Can you work these out from the model? Positions are in its coordinate system, mm. Face numbers are marked on the shaded views. A direction names the side the tool comes from. Give positions to 0.01 mm unless a question says otherwise; leave off trailing zeros. Loops run counter-clockwise (first coordinate to the right, second up) from the corner with the lowest first, then second, coordinate; pieces in that order, holes last. Notation, with made-up numbers: M -16.5,74.25 L 2.5,74.25 A25 ccw 2.5,101.25 Z; hole C -38.5,77 d1. An arc over 180 degrees is marked long. Put each result on its own line as item: value. Start each with the question number.
1) Imagine slicing it at C-C (x = -2). Write out the boundary of the cut face in (y, z), then the cut area to 3 significant figures.
2) For P1, Ø3.5, axis at x = 17, z = -1, coming from the +Y side; P2, Ø1.5, axis at x = 3, z = -2.5, coming from the +Y side; P3, Ø1.2, axis at x = -10, z = 6, coming from the +Y side, each with a flat end and sliding along its axis, tell me the tip position at first contact or that it passes through.
3) For the marked faces 4 and 5, which set-ups out of +Z, -Z, +X, -X, +Y, -Y let a thin tool reach every point of the face, with its end or its side?
4) Imagine slicing it at B-B (x = -18). Write out the boundary of the cut face in (y, z).
5) Imagine slicing it at A-A (z = 0). Write out the boundary of the cut face in (x, y), then the cut area to 3 significant figures.
6) If we mould it in two halves opening along X, with no side actions, what happens to the marked faces 1, 2 and 3? For each: +X half, -X half, draft (parallel to the pull), parting line (faces both ways), or undercut.
7) Please list where these lines run through material, in increasing order: line 1 along Y through (x, z) = (-2, 3.5); line 2 along Y through (x, z) = (12, 2.75). Write a range as from..to.
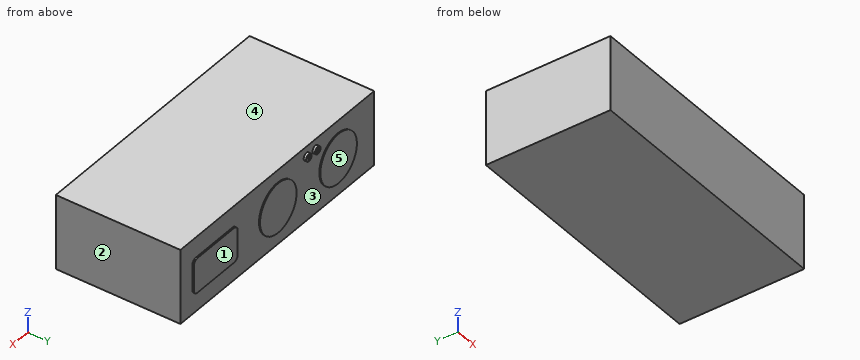
from build123d import *

# Parameters (mm, degrees)
SKETCH_1_W      = 53
SKETCH_1_H      = 15
EXTRUDE_1_DEPTH = 25
SKETCH_2_R      = 5
EXTRUDE_2_DEPTH = 0.2
SKETCH_3_R      = 0.75
EXTRUDE_4_DEPTH = 0.5
SKETCH_4_W      = 0.308010804
SKETCH_4_H      = 1.227700604
EXTRUDE_5_DEPTH = 0.3
SKETCH_6_W      = 0.300930155
SKETCH_6_H      = 1.191236652
EXTRUDE_8_DEPTH = 0.3
SKETCH_8_W      = 12
SKETCH_8_H      = 7
EXTRUDE_9_DEPTH = 0.3
FILLET_1_R      = 1
FILLET_2_R      = 1


with BuildPart() as part:
    # 草圖1 → 填料-伸長1 (new body)
    with BuildSketch(Plane(origin=(0, 0, 0), x_dir=(1, 0, 0), z_dir=(0, 1, 0))):
        Rectangle(SKETCH_1_W, SKETCH_1_H)
    extrude(amount=EXTRUDE_1_DEPTH)

    # 草圖2 → 填料-伸長2 (add)
    with BuildSketch(Plane(origin=(0, 25, 0), x_dir=(1, 0, 0), z_dir=(0, 1, 0))):
        with Locations(Location((0, 0, 0), (0, 0, 270))):
            Circle(SKETCH_2_R)
        with Locations(Location((-16.5, 0, 0), (0, 0, 270))):
            Circle(SKETCH_2_R)
    extrude(amount=EXTRUDE_2_DEPTH)

    # 草圖3 → 填料-伸長4 (add)
    with BuildSketch(Plane(origin=(0, 25, 0), x_dir=(1, 0, 0), z_dir=(0, 1, 0))):
        with Locations(Location((-7.968179653, -5.500848642, 0), (0, 0, 270))):
            Circle(SKETCH_3_R)
        with Locations(Location((-10.399702952, -5.500848642, 0), (0, 0, 270))):
            Circle(SKETCH_3_R)
    extrude(amount=EXTRUDE_4_DEPTH)

    # 草圖4 → 填料-伸長5 (add)
    with BuildSketch(Plane(origin=(0, 25.5, 0), x_dir=(1, 0, 0), z_dir=(0, 1, 0))):
        with Locations((-7.986543435, -5.513019863)):
            Rectangle(SKETCH_4_W, SKETCH_4_H)
    extrude(amount=EXTRUDE_5_DEPTH)

    # 草圖6 → 填料-伸長8 (add)
    with BuildSketch(Plane(origin=(0, 25.5, 0), x_dir=(1, 0, 0), z_dir=(0, 1, 0))):
        with Locations((-10.389863122, -5.481431278)):
            Rectangle(SKETCH_6_W, SKETCH_6_H)
    extrude(amount=EXTRUDE_8_DEPTH)

    # 草圖8 → 填料-伸長9 (add)
    with BuildSketch(Plane(origin=(0, 25, 0), x_dir=(1, 0, 0), z_dir=(0, 1, 0))):
        with Locations((17.250728111, 0.094744835)):
            Rectangle(SKETCH_8_W, SKETCH_8_H)
    extrude(amount=EXTRUDE_9_DEPTH)

    # 圓角1
    fillet_1_edges = [part.edges().sort_by_distance(p)[0] for p in [
        (23.250728111, 25.15, 3.405255165),
        (23.250728111, 25.15, -3.594744835),
        (11.250728111, 25.15, -3.594744835),
        (11.250728111, 25.15, 3.405255165),
    ]]
    fillet(fillet_1_edges, radius=FILLET_1_R)

    # 圓角2
    # the kernel refuses this fillet: 1 mm, written as the material it takes off along each edge
    with BuildSketch(Plane(origin=(-8.454040937, 25.8, 4.885812952), x_dir=(0, -1, 0), z_dir=(-1, 0, 0)), Plane(origin=(-12.325685306, 25.8, 6.077049604), x_dir=(0, -1, 0), z_dir=(1, 0, 0))) as fillet_2_piece_1:
        with BuildLine():
            CenterArc((1, 0.714142843), FILLET_2_R, 180, 45.572995999)
            Line((0, 0.714142843), (-0.02, 0.714142843))
            Line((-0.02, 0.714142843), (-0.02, 0))
            Line((-0.02, 0), (0, -0.02))
            ThreePointArc((0, -0.02), (0.15, -0.02), (0.286, -0.014282857))
            Line((0.286, -0.014282857), (0.3, 0))
        make_face()
    extrude(amount=3.871644369, mode=Mode.SUBTRACT)
    with BuildSketch(Plane(origin=(-9.925905944, 25.8, 6.126870165), x_dir=(0, -1, 0), z_dir=(1, 0, 0)), Plane(origin=(-6.047180926, 25.8, 4.899169561), x_dir=(0, -1, 0), z_dir=(-1, 0, 0))) as fillet_2_piece_2:
        with BuildLine():
            CenterArc((1, 0.714142843), FILLET_2_R, 180, 45.572995999)
            Line((0, 0.714142843), (-0.02, 0.714142843))
            Line((-0.02, 0.714142843), (-0.02, 0))
            Line((-0.02, 0), (0, -0.02))
            ThreePointArc((0, -0.02), (0.15, -0.02), (0.286, -0.014282857))
            Line((0.286, -0.014282857), (0.3, 0))
        make_face()
    extrude(amount=3.878725018, mode=Mode.SUBTRACT)


solid = part.part
Recorded:
1. outline: M 0,-7.5 L 25,-7.5 L 25,-4.58 L 25.2,-4.58 L 25.2,4.58 L 25,4.58 L 25,7.5 L 0,7.5 Z
1. area: 377 mm²
2. P1: y = 25.3
2. P2: y = 25.2
2. P3: y = 25.79
3. face 4: +Z, +X, -X, +Y, -Y
3. face 5: +Z, -Z, -X, +Y
4. outline: M 0,-7.5 L 25,-7.5 L 25,-4.77 L 25.2,-4.77 L 25.2,4.77 L 25,4.77 L 25,7.5 L 0,7.5 Z
5. outline: M -26.5,0 L 26.5,0 L 26.5,25 L 23.25,25 L 23.25,25.3 L 11.25,25.3 L 11.25,25 L 5,25 L 5,25.2 L -5,25.2 L -5,25 L -11.5,25 L -11.5,25.2 L -21.5,25.2 L -21.5,25 L -26.5,25 Z
5. area: 1,330 mm²
6. face 1: draft
6. face 2: +X half
6. face 3: undercut
7. line 1: 0..25.2
7. line 2: 0..25.3
